Geometry: final body of the model. Coordinates: model frame, mm. A direction names the side the tool comes from. Coordinates: 2 decimals unless noted, no trailing zeros. Loops run counter-clockwise (first coordinate to the right, second up) from the corner with the lowest first, then second, coordinate; pieces in that order, holes last. Notation, with made-up numbers: (-40, 67.25) - (-7, 67.25) arc R18 cw to (-7, 97.25) - close; hole circle Ø2 at (74.5, 74.25). An arc over 180 degrees is marked (long way). Put each result on its own line as item: value. Start each with the question number.
1) Contact query for flat-ended pins moving along their axis: pin 1 Ø8 at (x, z) = (35, 13) entering from +Y; pin 2 Ø1 at (x, z) = (-16, -25) entering from -Y; pin 3 Ø1.3 at (y, z) = (88.5, -9) entering from +X. Output: stop coordinate, or through.
2) Material intervals for line 1 along X through (y, z) = (65, 6.5); line 2 along X through (y, z) = (1.3, 0), sorted ascending. Write a range as from..to.
3) Reachability of faces 1 (the flat face through (48, 49, 1)), 2 (the flat face through (-28, 43, 49)), 3 (the flat face through (-49, 19, 31)) from +Z, -Z, +X, -X, +Y, -Y: full face, straight path, thin tool, end or side. Return the list, or none.
4) Section B-B on x = 5. Output: boundary loops of the cut face in (y, z), and give its area (3 significant figures).
5) Draft query along Y for faces 4 (the flat face through (-49, 84, -40)), 5 (the flat face through (-1, 49, -48)). Return one class per face: +Y half, -Y half, draft (parallel to the pull), parting line (faces both ways), or undercut.
6) Section A-A on z = -27.5. Output: boundary loops of the cut face in (x, y), and give its area (3 significant figures).
```python
from build123d import *

# Parameters (mm, degrees)
IZIM1_W                     = 100
IZIM1_H                     = 100
IZIM1_R                     = 24.5
Y_KSEKLIK_EKSTR_ZYON1_DEPTH = 2
IZIM2_W                     = 100
IZIM2_H                     = 100
IZIM2_W_2                   = 96
IZIM2_H_2                   = 96
Y_KSEKLIK_EKSTR_ZYON2_DEPTH = 96
IZIM3_W                     = 6.808697121
IZIM3_H                     = 2.995826734
IZIM3_W_2                   = 3.540522504
IZIM3_H_2                   = 13.072698474
IZIM3_W_3                   = 8.715132316
IZIM3_W_4                   = 9.959144329
IZIM3_H_3                   = 3.786659795
IZIM3_W_5                   = 6.536349237
IZIM3_H_4                   = 5.991653467
IZIM3_W_6                   = 4.357566158
IZIM3_H_5                   = 3.268174619
IZIM3_H_6                   = 5.446957697
IZIM3_H_7                   = 1.63408731
KES_EKSTR_ZYON1_DEPTH       = 1
IZIM4_W                     = 2.855123206
IZIM4_H                     = 4.861170012
IZIM4_W_2                   = 11.319008014
IZIM4_H_2                   = 1.730473094
IZIM4_W_3                   = 2.714479197
IZIM4_H_3                   = 10.322809225
IZIM4_W_4                   = 9.387113738
IZIM4_H_4                   = 3.377434488
IZIM4_W_5                   = 4.989274294
IZIM4_H_5                   = 13.829779239
IZIM4_W_6                   = 7.288706005
IZIM4_H_6                   = 5.901605045
IZIM4_W_7                   = 5.357045211
IZIM4_H_7                   = 5.315156672
IZIM4_W_8                   = 2.340389822
IZIM4_H_8                   = 9.060236987
KES_EKSTR_ZYON2_DEPTH       = 1
IZIM5_W                     = 2.995826734
IZIM5_H                     = 4.357566158
IZIM5_W_2                   = 11.16626328
IZIM5_H_2                   = 1.634087309
IZIM5_W_3                   = 2.995826733
IZIM5_H_3                   = 7.625740777
IZIM5_W_4                   = 7.353392891
IZIM5_W_5                   = 3.812870388
IZIM5_H_4                   = 8.442784431
IZIM5_W_6                   = 8.987480201
IZIM5_H_5                   = 2.451130964
IZIM5_W_7                   = 3.268174618
IZIM5_H_6                   = 6.264001352
KES_EKSTR_ZYON3_DEPTH       = 1
IZIM6_W                     = 2.982026027
IZIM6_H                     = 8.051470273
IZIM6_W_2                   = 11.033496299
IZIM6_H_2                   = 1.789215616
IZIM6_W_3                   = 2.385620822
IZIM6_H_3                   = 9.840685888
IZIM6_W_4                   = 7.455065067
IZIM6_H_4                   = 2.385620821
IZIM6_W_5                   = 12.822711915
IZIM6_H_5                   = 2.982026027
IZIM6_H_6                   = 5.069444246
IZIM6_W_6                   = 3.876633835
IZIM6_H_7                   = 6.858659862
IZIM6_W_7                   = 4.473039041
IZIM6_H_8                   = 8.647875478
KES_EKSTR_ZYON4_DEPTH       = 1


with BuildPart() as part:
    # Çizim1 → Yükseklik-Ekstrüzyon1 (new body)
    with BuildSketch(Plane(origin=(0, 0, 0), x_dir=(1, 0, 0), z_dir=(0, 1, 0))):
        Rectangle(IZIM1_W, IZIM1_H)
        with Locations(Location((0, 0, 0), (0, 0, 270))):
            Circle(IZIM1_R, mode=Mode.SUBTRACT)
    extrude(amount=Y_KSEKLIK_EKSTR_ZYON1_DEPTH)

    # Çizim2 → Yükseklik-Ekstrüzyon2 (add)
    with BuildSketch(Plane(origin=(0, 2, 0), x_dir=(1, 0, 0), z_dir=(0, 1, 0))):
        Rectangle(IZIM2_W, IZIM2_H)
        Rectangle(IZIM2_W_2, IZIM2_H_2, mode=Mode.SUBTRACT)
    extrude(amount=Y_KSEKLIK_EKSTR_ZYON2_DEPTH)

    # Çizim3 → Kes-Ekstrüzyon1 (cut)
    with BuildSketch(Plane.XY.offset(50)):
        with Locations((-38.128703883, 80.524267674)):
            Rectangle(IZIM3_W, IZIM3_H)
        with Locations((-6.808697122, 60.642872078)):
            Rectangle(IZIM3_W_2, IZIM3_H_2)
        with Locations((-27.643310315, 43.348781389)):
            Rectangle(IZIM3_W_3, IZIM3_H)
        with Locations((21.106961078, 60.642872079)):
            Rectangle(IZIM3_W_4, IZIM3_H_3)
        with Locations((21.106961078, 25.50999493)):
            Rectangle(IZIM3_W_5, IZIM3_H_4)
        with Locations((-12.119480877, 15.569297132)):
            Rectangle(IZIM3_W_6, IZIM3_H_5)
        with Locations((12.255654819, 11.484078859)):
            Rectangle(IZIM3_W_6, IZIM3_H_6)
        with Locations((21.106961078, 86.379747199)):
            Rectangle(IZIM3_W_4, IZIM3_H_7)
    extrude(amount=-KES_EKSTR_ZYON1_DEPTH, mode=Mode.SUBTRACT)

    # Çizim4 → Kes-Ekstrüzyon2 (cut)
    with BuildSketch(Plane.ZY.offset(50)):
        with Locations((-40.12319253, 84.166167132)):
            Rectangle(IZIM4_W, IZIM4_H)
        with Locations((0, 48.061123669)):
            Rectangle(IZIM4_W_2, IZIM4_H_2)
        with Locations((12.386939179, 68.745292742)):
            Rectangle(IZIM4_W_3, IZIM4_H_3)
        with Locations((26.279902445, 54.531767203)):
            Rectangle(IZIM4_W_4, IZIM4_H_4)
        with Locations((-26.801088585, 31.592223885)):
            Rectangle(IZIM4_W_5, IZIM4_H_5)
        with Locations((7.385346578, 16.750764677)):
            Rectangle(IZIM4_W_6, IZIM4_H_6)
        with Locations((30.973459314, 18.564160483)):
            Rectangle(IZIM4_W_7, IZIM4_H_7)
        with Locations((-17.619740697, 72.897531843)):
            Rectangle(IZIM4_W_8, IZIM4_H_8)
    extrude(amount=-KES_EKSTR_ZYON2_DEPTH, mode=Mode.SUBTRACT)

    # Çizim5 → Kes-Ekstrüzyon3 (cut)
    with BuildSketch(Plane(origin=(0, 0, -50), x_dir=(-1, 0, 0), z_dir=(0, 0, -1))):
        with Locations((-29.822093394, 73.443222668)):
            Rectangle(IZIM5_W, IZIM5_H)
        with Locations((-6.944871064, 67.179221316)):
            Rectangle(IZIM5_W_2, IZIM5_H_2)
        with Locations((25.056005409, 45.799912353)):
            Rectangle(IZIM5_W_3, IZIM5_H_3)
        with Locations((6.12782741, 31.773996282)):
            Rectangle(IZIM5_W_4, IZIM5_H)
        with Locations((-28.324180027, 21.969472427)):
            Rectangle(IZIM5_W_5, IZIM5_H_4)
        with Locations((25.056005408, 16.250166844)):
            Rectangle(IZIM5_W_6, IZIM5_H_5)
        with Locations((18.928177999, 78.754006423)):
            Rectangle(IZIM5_W_7, IZIM5_H_6)
    extrude(amount=-KES_EKSTR_ZYON3_DEPTH, mode=Mode.SUBTRACT)

    # Çizim6 → Kes-Ekstrüzyon4 (cut)
    with BuildSketch(Plane(origin=(50, 0, 0), x_dir=(0, 0, -1), z_dir=(1, 0, 0))):
        with Locations((-33.547792801, 75.286818133)):
            Rectangle(IZIM6_W, IZIM6_H)
        with Locations((-8.349672875, 62.76230882)):
            Rectangle(IZIM6_W_2, IZIM6_H_2)
        with Locations((31.758577185, 37.862391497)):
            Rectangle(IZIM6_W_3, IZIM6_H_3)
        with Locations((32.951387596, 71.261082997)):
            Rectangle(IZIM6_W_4, IZIM6_H_4)
        with Locations((-6.411355958, 27.574401705)):
            Rectangle(IZIM6_W_5, IZIM6_H_5)
        with Locations((-35.038805815, 13.111575475)):
            Rectangle(IZIM6_W, IZIM6_H_6)
        with Locations((21.17238479, 12.216967667)):
            Rectangle(IZIM6_W_6, IZIM6_H_7)
        with Locations((8.647875478, 87.960428746)):
            Rectangle(IZIM6_W_7, IZIM6_H_8)
    extrude(amount=-KES_EKSTR_ZYON4_DEPTH, mode=Mode.SUBTRACT)


solid = part.part
```
Answer block:
1. pin 1: stops at y = 2
1. pin 2: stops at y = 0
1. pin 3: stops at x = 49
2. line 1: x = -50..-48, 48..50
2. line 2: x = -50..-24.5, 24.5..50
3. face 1: +Y
3. face 2: +Z
3. face 3: -X
4. outline: (0, -50) - (66.36, -50) - (66.36, -49) - (68, -49) - (68, -50) - (98, -50) - (98, -48) - (2, -48) - (2, -23.98) - (0, -23.98) - close; (0, 23.98) - (2, 23.98) - (2, 48) - (98, 48) - (98, 50) - (0, 50) - close
4. area: 486 mm²
5. face 4: undercut
5. face 5: draft
6. outline: (-50, 0) - (50, 0) - (50, 98) - (48, 98) - (48, 2) - (-48, 2) - (-48, 98) - (-50, 98) - (-50, 38.51) - (-49, 38.51) - (-49, 24.68) - (-50, 24.68) - close
6. area: 570 mm²
